Could you check a few things on this model? Use its own coordinates, in mm. A direction names the side the tool comes from. Coordinates: 2 decimals unless noted, no trailing zeros. Loops run counter-clockwise (first coordinate to the right, second up) from the corner with the lowest first, then second, coordinate; pieces in that order, holes last. Notation, with made-up numbers: (-9.5, 31) -> (38.5, 31) arc R17 ccw to (38.5, 53) -> close; hole circle Ø5 at (83, 46.25). An arc over 180 degrees is marked (long way). One line per question, with ' | ' between items. Start each with the question number.
(1) Suppose I cut it at D-D (z = 8.5). Please give me the cut outline in (x, y).
(2) I'm going to push flat-ended pins straight in: pin 1 Ø2.5 at (x, z) = (-23.49, 5) entering from -Y; pin 2 Ø3 at (y, z) = (-14, 3.5) entering from -X; pin 3 Ø6 at (y, z) = (-7, 4) entering from -X; pin 4 Ø4 at (y, z) = (-7, 5) entering from +X. Where does each tip first touch, or does it pass through?
(3) If I drill on line 1 along Y through (x, z) = (0, 4.5); line 2 along Z through (x, y) = (22.5, 0.5); line 3 along X through (y, z) = (-9.75, 4.75), over which ranges is the centre line in solid material (lowest first)?
(4) If we mould it in two halves opening along X, with no side actions, what happens to faces 1 (the face through (-28.257, 1, 5)), 2 (the face through (21, 3, 5)), 3 (the face through (24.9, 1.5, 5.5))? For each: pulls with the +X half, pulls with the -X half, needs draft (parallel to the pull), parting line crosses it, or undercut.
(5) Which directions (+Z, -Z, +X, -X, +Y, -Y) give clear straight access to the entire face, cutting with the end or side of a thin tool? Please do faces 4 (the face through (-25.2, 0, 4.9)), 5 (the face through (-4, -17, 10)), 6 (the face through (25, 0, 4)).
(6) Suppose I cut it at C-C (y = -11.75). Please give me the cut outline in (x, z), plus the area to 3 significant figures.
(7) Suppose I cut it at B-B (x = 23). Please give me the cut outline in (y, z).
(8) Suppose I cut it at A-A (z = 5). Please give me the cut outline in (x, y), plus the area to 3 significant figures.
```python
from build123d import *

# Parameters (mm, degrees)
SKETCH1_W           = 1.27
SKETCH1_H           = 3
BOSS_EXTRUDE1_DEPTH = 10
CUT_EXTRUDE1_DEPTH  = 3


with BuildPart() as part:
    # Sketch1 → Boss-Extrude1 (new body)
    with BuildSketch(Plane.XY):
        with BuildLine():
            ThreePointArc((17.250000044, 0), (-1.505747486, -17.18415625), (-16.987127524, 3))
            Line((-16.987127524, 3), (-26.987127524, 3))
            Line((-26.987127524, 3), (-26.987127524, 0))
            Line((-26.987127524, 0), (-20.250000044, 0))
            ThreePointArc((-20.250000044, 0), (0, -20.250000044), (20.250000044, 0))
            Line((20.250000044, 0), (26.987127524, 0))
            Line((26.987127524, 0), (26.987127524, 3))
            Line((26.987127524, 3), (16.987127524, 3))
            ThreePointArc((16.987127524, 3), (17.18415625, 1.505747486), (17.250000044, 0))
        make_face()
        with Locations((27.622127524, 1.5)):
            Rectangle(SKETCH1_W, SKETCH1_H)
        with Locations((-27.622127524, 1.5)):
            Rectangle(SKETCH1_W, SKETCH1_H)
    extrude(amount=BOSS_EXTRUDE1_DEPTH)

    # Sketch2 → Cut-Extrude1 (cut)
    with BuildSketch(Plane(origin=(0, 3, 0), x_dir=(1, 0, 0), z_dir=(0, 1, 0))):
        with BuildLine():
            ThreePointArc((-21.987127524, -5), (-23.487127524, -3.5), (-24.987127524, -5))
            Line((-24.987127524, -5), (-21.987127524, -5))
        make_face()
        with BuildLine():
            Line((-21.987127524, -5), (-24.987127524, -5))
            ThreePointArc((-24.987127524, -5), (-23.487127524, -6.5), (-21.987127524, -5))
        make_face()
    cut_extrude1 = extrude(amount=-CUT_EXTRUDE1_DEPTH, mode=Mode.SUBTRACT)

    # Mirror1: Cut-Extrude1 across plane
    add(cut_extrude1.mirror(Plane(origin=(0, 0, 0), x_dir=(0, 0, 1), z_dir=(1, 0, 0))), mode=Mode.SUBTRACT)


solid = part.part
```
Checks:
1) outline: (-28.26, 0) -> (-20.25, 0) arc R20.25 ccw to (20.25, 0) -> (28.26, 0) -> (28.26, 3) -> (16.99, 3) arc R17.25 cw (long way) to (-16.99, 3) -> (-28.26, 3) -> close
2) pin 1: passes through | pin 2: stops at x = -15.93 | pin 3: stops at x = -19.85 | pin 4: stops at x = 19.62
3) line 1: y = -20.25 to -17.25 | line 2: z = 0 to 3.87, 6.13 to 10 | line 3: x = -17.75 to -14.23, 14.23 to 17.75
4) face 1: pulls with the -X half | face 2: needs draft | face 3: undercut
5) face 4: +Z, -Z, -X, -Y | face 5: +Z, +X, -X, +Y, -Y | face 6: +Z, -Z, +X, -Y
6) outline: (-16.49, 0) -> (-12.63, 0) -> (-12.63, 10) -> (-16.49, 10) -> close; (12.63, 0) -> (16.49, 0) -> (16.49, 10) -> (12.63, 10) -> close | area: 77.3 mm^2
7) outline: (0, 0) -> (3, 0) -> (3, 3.58) -> (0, 3.58) -> close; (0, 6.42) -> (3, 6.42) -> (3, 10) -> (0, 10) -> close
8) outline: (-28.26, 0) -> (-24.99, 0) -> (-24.99, 3) -> (-28.26, 3) -> close; (-21.99, 0) -> (-20.25, 0) arc R20.25 ccw to (20.25, 0) -> (21.99, 0) -> (21.99, 3) -> (16.99, 3) arc R17.25 cw (long way) to (-16.99, 3) -> (-21.99, 3) -> close; (24.99, 0) -> (28.26, 0) -> (28.26, 3) -> (24.99, 3) -> close | area: 225 mm^2
